```python
from build123d import *

# Parameters (mm, degrees)
SKETCH1_W           = 20
SKETCH1_H           = 132
BOSS_EXTRUDE1_DEPTH = 3
SKETCH2_W           = 20
SKETCH2_H           = 5
BOSS_EXTRUDE2_DEPTH = 67
SKETCH4_R           = 1.875
CUT_EXTRUDE1_DEPTH  = 150.746452379
FILLET3_R           = 10
CUT_EXTRUDE2_DEPTH  = 3.5
CUT_EXTRUDE3_DEPTH  = 3.5
SKETCH8_W           = 45
SKETCH8_H           = 20
BOSS_EXTRUDE3_DEPTH = 3
CHAMFER1_SIZE       = 5
FILLET4_R           = 10
FILLET5_R           = 4
FILLET6_R           = 20


# Some blends are built 0.0001 mm under size
with BuildPart() as part:
    # Sketch1 → Boss-Extrude1 (new body)
    with BuildSketch(Plane(origin=(0, 0, 0), x_dir=(1, 0, 0), z_dir=(0, 1, 0))):
        Rectangle(SKETCH1_W, SKETCH1_H)
    extrude(amount=BOSS_EXTRUDE1_DEPTH)

    # Sketch2 → Boss-Extrude2 (add)
    with BuildSketch(Plane(origin=(0, 3, 0), x_dir=(1, 0, 0), z_dir=(0, 1, 0))):
        with Locations((0, -63.5)):
            Rectangle(SKETCH2_W, SKETCH2_H)
        with Locations((0, 63.5)):
            Rectangle(SKETCH2_W, SKETCH2_H)
    extrude(amount=BOSS_EXTRUDE2_DEPTH)

    # Sketch4 → Cut-Extrude1 (cut, through all)
    with BuildSketch(Plane.XY.offset(66)):
        with Locations((0, 65.2375)):
            Circle(SKETCH4_R)
    extrude(amount=-CUT_EXTRUDE1_DEPTH, mode=Mode.SUBTRACT)

    # Fillet3
    fillet3_edges = [part.edges().sort_by_distance(p)[0] for p in [
        (10, 70, 63.5),
        (-10, 70, 63.5),
        (10, 70, -63.5),
        (-10, 70, -63.5),
    ]]
    fillet(fillet3_edges, radius=FILLET3_R - 0.0001)  # a hair under: the kernel refuses the full size

    # Sketch6 → Cut-Extrude2 (cut)
    with BuildSketch(Plane.XY.offset(66)):
        Polygon((3.175426481, 65.2375), (1.58771324, 67.9875), (-1.58771324, 67.9875), (-3.175426481, 65.2375), (-1.58771324, 62.4875), (1.58771324, 62.4875), align=None)
    extrude(amount=-CUT_EXTRUDE2_DEPTH, mode=Mode.SUBTRACT)

    # Sketch7 → Cut-Extrude3 (cut)
    with BuildSketch(Plane(origin=(0, 0, -66), x_dir=(-1, 0, 0), z_dir=(0, 0, -1))):
        Polygon((3.175426481, 65.2375), (1.58771324, 67.9875), (-1.58771324, 67.9875), (-3.175426481, 65.2375), (-1.58771324, 62.4875), (1.58771324, 62.4875), align=None)
    extrude(amount=-CUT_EXTRUDE3_DEPTH, mode=Mode.SUBTRACT)

    # Sketch8 → Boss-Extrude3 (add)
    with BuildSketch(Plane.XZ):
        Polygon((17.5, -56), (17.5, -66), (-17.5, -66), (-17.5, -56), (-10, -31), (10, -31), align=None)
        Polygon((17.5, 56), (17.5, 66), (-17.5, 66), (-17.5, 56), (-10, 31), (10, 31), align=None)
        with Locations((22.5, 0)):
            Rectangle(SKETCH8_W, SKETCH8_H)
    extrude(amount=-BOSS_EXTRUDE3_DEPTH)

    # Chamfer1
    chamfer1_edges = [part.edges().sort_by_distance(p)[0] for p in [
        (10, 3, -63.5),
        (-10, 3, -63.5),
        (10, 3, 63.5),
        (-10, 3, 63.5),
        (0, 3, 61),
        (0, 3, -61),
    ]]
    chamfer(chamfer1_edges, length=CHAMFER1_SIZE)

    # Fillet4
    fillet4_edges = [part.edges().sort_by_distance(p)[0] for p in [
        (45, 1.5, -10),
        (45, 1.5, 10),
    ]]
    fillet(fillet4_edges, radius=FILLET4_R - 0.0001)  # a hair under: the kernel refuses the full size

    # Fillet5
    fillet5_edges = [part.edges().sort_by_distance(p)[0] for p in [
        (17.5, 1.5, -66),
        (-17.5, 1.5, -66),
        (-17.5, 1.5, 66),
        (17.5, 1.5, 66),
    ]]
    fillet(fillet5_edges, radius=FILLET5_R)

    # Fillet6
    # the kernel refuses this fillet: 20 mm, written as the material it adds along each edge
    with BuildSketch(Plane(origin=(-10, 0, -31), x_dir=(-0.287347885566345, 0, -0.9578262852211515), z_dir=(0, 1, 0)), Plane(origin=(-10, 0, 31), x_dir=(0, 0, -1), z_dir=(0, 1, 0))) as fillet6_piece_1:
        with BuildLine():
            CenterArc((FILLET6_R * 0.146768836304, FILLET6_R), FILLET6_R, 253.300755766, 16.699244234)
            Line((-FILLET6_R * 0.140579049263, FILLET6_R * 0.0421737147788), (0, 0))
            Line((0, 0), (FILLET6_R * 0.146768836304, 0))
        make_face()
    extrude(amount=3)
    with BuildSketch(Plane(origin=(10, 0, 31), x_dir=(0, 0, -1), z_dir=(0, 1, 0)), Plane(origin=(10, 0, -31), x_dir=(0.287347885566345, 0, -0.9578262852211515), z_dir=(0, 1, 0))) as fillet6_piece_2:
        with BuildLine():
            CenterArc((FILLET6_R * 0.146768836304, -FILLET6_R), FILLET6_R, 90, 16.699244234)
            Line((-FILLET6_R * 0.140579049263, -FILLET6_R * 0.0421737147788), (0, 0))
            Line((0, 0), (FILLET6_R * 0.146768836304, 0))
        make_face()
    extrude(amount=3)
    with BuildSketch(Plane(origin=(10, 3, -10), x_dir=(0, 0, -1), z_dir=(0, -1, 0))) as fillet6_piece_3:
        with BuildLine():
            CenterArc((FILLET6_R, FILLET6_R), FILLET6_R, 180, 90)
            Line((0, FILLET6_R), (0, 0))
            Line((0, 0), (FILLET6_R, 0))
        make_face()
    extrude(amount=3)
    with BuildSketch(Plane(origin=(10, 0, 10), x_dir=(1, 0, 0), z_dir=(0, 1, 0))) as fillet6_piece_4:
        with BuildLine():
            CenterArc((FILLET6_R, -FILLET6_R), FILLET6_R, 90, 90)
            Line((0, -FILLET6_R), (0, 0))
            Line((0, 0), (FILLET6_R, 0))
        make_face()
    extrude(amount=3)


solid = part.part
```
Here's how the part is built. I have some questions about the finished solid (model axes, mm). A direction names the side the tool comes from. Give positions to 0.01 mm unless a question says otherwise; leave off trailing zeros. Order: outer loops, then holes, each group sorted by start corner. A loop starts at its lowest first (then second) coordinate and runs counter-clockwise, first axis right, second up. Notation, with made-up numbers: M -26,-36 L -13,-36 A4 cw -13,-31 Z; hole C -9,4.5 d11. An arc over 180 degrees is marked long. Use a Markdown table: item, result. Add a question column.
1. If we mould it in two halves opening along Z, with no side actions, what happens to faces 5 (the flat face through (32, 1, 10)), 6 (the cylindrical face through (16.359, 1.781, -64.797)), 7 (the flat face through (-10, 1, 0))? For each: +Z half, -Z half, draft (parallel to the pull), parting line (faces both ways), or undercut.
2. On a 3-axis mill with a long thin cutter (end or side, diameter ignored), from which of +Z, -Z, +X, -X, +Y, -Y can I reach the whole of each face in a straight line? I mean faces 1 (the flat face through (-10, 34, 64)), 2 (the flat face through (10, 34, 64)), 3 (the flat face through (14.125, 1.479, -44.75)), 4 (the cylindrical face through (-10.22, 1.48, 31.01)). Say none if no direction works.
3. Suppose I cut it at B-B (z = -46). List the corners of the cut face in (x, y) for me.
4. Suppose I cut it at C-C (x = -8). List the corners of the cut face in (y, z) for me, and give its area (3 significant figures).
5. Suppose I cut it at A-A (y = 30). List the corners of the cut face in (x, z) for me.
6. For pin 1 Ø3.5 at (y, z) = (2, -58) entering from +X; pin 2 Ø8 at (x, z) = (1, -26.5) entering from +Y; pin 3 Ø5 at (x, y) = (0, 65.24) entering from -Z, each with a flat end and sliding along its axis, tell me the tip position at first contact or that it passes through.
7. I need wall thicknesses on probe 1 along Z at (x, y) = (0, 24); probe 2 along Y at (x, z) = (0, -61.9); probe 3 along Y at (x, z) = (1, -32). Which ranges of each line are inside material? Lowest first, please. Write a range as from..to.
8. Suppose I cut it at D-D (z = 45). List the corners of the cut face in (x, y) for me.
Results list:
| question | item | result |
|---|---|---|
| 1 | face 5 | +Z half |
| 1 | face 6 | -Z half |
| 1 | face 7 | undercut |
| 2 | face 1 | +Z, -Z, -X, +Y |
| 2 | face 2 | +Z, -Z, +X, +Y |
| 2 | face 3 | +X, +Y, -Y |
| 2 | face 4 | -X, +Y, -Y |
| 3 | outline | M -14.5,0 L 14.5,0 L 14.5,3 L -14.5,3 Z |
| 4 | outline | M 0,-66 L 66,-66 L 66,-61 L 8,-61 L 3,-56 L 3,56 L 8,61 L 66,61 L 66,66 L 0,66 Z |
| 4 | area | 1,050 mm² |
| 5 | outline | M -10,-66 L 10,-66 L 10,-61 L -10,-61 Z; M -10,61 L 10,61 L 10,66 L -10,66 Z |
| 6 | pin 1 | stops at x = 17.5 |
| 6 | pin 2 | stops at y = 3 |
| 6 | pin 3 | stops at z = -62.5 |
| 7 | probe 1 | z = -66..-61, 61..66 |
| 7 | probe 2 | y = 0..63.36, 67.11..70 |
| 7 | probe 3 | y = 0..3 |
| 8 | outline | M -14.2,0 L 14.2,0 L 14.2,3 L -14.2,3 Z |
